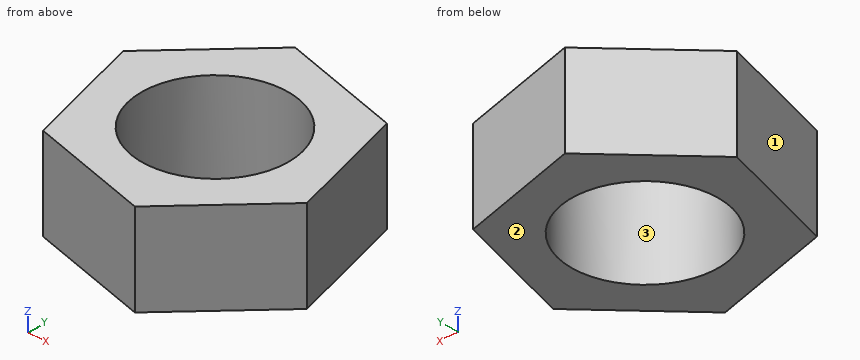
from build123d import *

# Parameters (mm, degrees)
CROQUIS1_R              = 6
CROQUIS1_R_2            = 2.5
SALIENTE_EXTRUIR1_DEPTH = 5
CROQUIS2_R              = 4
SALIENTE_EXTRUIR2_DEPTH = 5
CROQUIS3_R              = 4
CORTAR_EXTRUIR1_DEPTH   = 10


with BuildPart() as part:
    # Croquis1 → Saliente-Extruir1 (new body)
    with BuildSketch(Plane.XY):
        Circle(CROQUIS1_R)
        Circle(CROQUIS1_R_2, mode=Mode.SUBTRACT)
    extrude(amount=SALIENTE_EXTRUIR1_DEPTH)

    # Croquis2 → Saliente-Extruir2 (add)
    with BuildSketch(Plane.XY.offset(5)):
        Polygon((-6.692111353, 1.79322214), (-1.793079748, 6.692149506), (4.899031604, 4.898927366), (6.692111353, -1.79322214), (1.793079748, -6.692149506), (-4.899031604, -4.898927366), align=None)
        Circle(CROQUIS2_R, mode=Mode.SUBTRACT)
    extrude(amount=-SALIENTE_EXTRUIR2_DEPTH)

    # Croquis3 → Cortar-Extruir1 (cut)
    with BuildSketch(Plane.XY.offset(5)):
        Circle(CROQUIS3_R)
    extrude(amount=-CORTAR_EXTRUIR1_DEPTH, mode=Mode.SUBTRACT)


solid = part.part
Could you check a few things on this model? Use its own coordinates, in mm. Face numbers are marked on the shaded views. Round coordinates to 2 decimals unless told otherwise and drop trailing zeros. Loops run counter-clockwise (first coordinate to the right, second up) from the corner with the lowest first, then second, coordinate; pieces in that order, holes last. Notation, with made-up numbers: (-36.5, 50.25) - (16.5, 50.25) arc R23 ccw to (16.5, 60.25) - close; hole circle Ø1 at (-21.5, 31). An arc over 180 degrees is marked (long way). Write item = value, one per line.
1) I need wall thicknesses on line 1 along Y through (x, z) = (-2, 1.9); line 2 along X through (y, z) = (3, 3.4); line 3 along Y through (x, z) = (0, 2.35). Which ranges of each line are inside material? Lowest first, please. Write a range as from..to.
Computed:
line_1 = -5.68..-3.46, 3.46..6.49
line_2 = -5.49..-2.65, 2.65..5.41
line_3 = -6.21..-4, 4..6.21
2) Imagine slicing it at D-D (x = 5.25). Please give me the cut outline in (y, z), and give its area (3 significant figures).
Computed:
outline = (-3.24, 0) - (3.59, 0) - (3.59, 5) - (-3.24, 5) - close
area = 34.1 mm2
3) Imagine slicing it at A-A (z = 2.1). Please give me the cut outline in (x, y).
Computed:
outline = (-6.69, 1.79) - (-4.9, -4.9) - (1.79, -6.69) - (6.69, -1.79) - (4.9, 4.9) - (-1.79, 6.69) - close; hole circle Ø8 at (0, 0)
4) I'm going to push flat-ended pins straight in: P1, Ø3, axis at x = 4, y = 0, coming from the -Z side; P2, Ø1.5, axis at y = 3, z = 3.5, coming from the -X side. Where does each tip first touch, or does it pass through?
Computed:
P1 = 0
P2 = -6.24
5) Imagine slicing it at B-B (x = 1). Please give me the cut outline in (y, z), and give its area (3 significant figures).
Computed:
outline = (-6.48, 0) - (-3.87, 0) - (-3.87, 5) - (-6.48, 5) - close; (3.87, 0) - (5.94, 0) - (5.94, 5) - (3.87, 5) - close
area = 23.4 mm2
6) If we mould it in two halves opening along Y, with no side actions, what happens to the marked faces 1, 2 and 3? For each: pulls with the +Y half, pulls with the -Y half, needs draft (parallel to the pull), parting line crosses it, or undercut.
Computed:
face_1 = pulls with the -Y half
face_2 = needs draft
face_3 = undercut
7) Imagine slicing it at C-C (y = -3.5). Please give me the cut outline in (x, z).
Computed:
outline = (-5.27, 0) - (-1.94, 0) - (-1.94, 5) - (-5.27, 5) - close; (1.94, 0) - (4.99, 0) - (4.99, 5) - (1.94, 5) - close
